The listing builds one solid part. Answer for the finished solid, in the listing's coordinates (mm). A direction names the side the tool comes from. Coordinates: 2 decimals unless noted, no trailing zeros. Loops run counter-clockwise (first coordinate to the right, second up) from the corner with the lowest first, then second, coordinate; pieces in that order, holes last. Notation, with made-up numbers: (58, 58) - (70, 58) arc R15 cw to (70, 73) - close; hole circle Ø9 at (-29, 86). An arc over 180 degrees is marked (long way). Return JSON: item names as keys, results as strings. Group by question number.
1. Each of these flat-tipped pins is pushed along its axis until it touches: P1, Ø3, axis at x = -6, y = 64, coming from the +Z side; P2, Ø1.5, axis at y = 56.5, z = -9, coming from the +X side; P3, Ø10.5, axis at x = -42, z = -24, coming from the +Y side; P4, Ø6, axis at x = 42, z = -6, coming from the +Y side. Where does it stop, or does it pass through?
2. Section D-D (x = -30) is taken. Write down the section's boundary in (y, z), and give its area (3 significant figures).
3. The mould has two halves that part along Y. Classify faces 4 (the face through (-38, 10, -15)), 5 (the face through (25, 51, -15)), 6 (the face through (-0.465, 27.507, -7.395)): pulls with the +Y half, pulls with the -Y half, needs draft (parallel to the pull), parting line crosses it, or undercut.
4. Section C-C (y = 42.5) is taken. Write down the section's boundary in (x, z).
5. Which of the six approach directions +Z, -Z, +X, -X, +Y, -Y give full straight-line access (tool end or side, diameter ignored) to faces 1 (the face through (-23.938, 25.702, -14.79)), 2 (the face through (23.938, 25.702, -14.79)), 3 (the face through (-39.381, 4.585, -21.992))?
6. Section A-A (z = -24) is taken. Write down the section's boundary in (x, y), and give its area (3 significant figures).
7. Section B-B (x = 42) is taken. Write down the section's boundary in (y, z), and give its area (3 significant figures).
8. Find the intervals of material crossed by line 1 along X through (y, z) = (6, -24); line 2 along Z through (x, y) = (42, 4.75); line 3 along Y through (x, z) = (0, -25.75), in increasing order.
```python
from build123d import *

# Parameters (mm, degrees)
EXTRUDE_1_DEPTH             = 30
SKETCH_2_R                  = 20
CUT_EXTRUDE_1_DEPTH         = 15
SKETCH_3_R                  = 5
CUT_EXTRUDE_2_DEPTH         = 109.397550478
FILLET_5_R                  = 6
SKETCH_4_R                  = 15
CUT_EXTRUDE_3_DEPTH         = 15
FILLET_6_R                  = 2
HOLE_WIZARD_M62_D           = 6.6
HOLE_WIZARD_M62_CSINK_D     = 8
HOLE_WIZARD_M62_CSINK_ANGLE = 90
PATTERN_LINEAR_1_COUNT      = 2
PATTERN_LINEAR_1_PITCH      = 18
PATTERN_LINEAR_1_COUNT_DIR2 = 2
PATTERN_LINEAR_1_PITCH_DIR2 = 84
FILLET_7_R                  = 3


with BuildPart() as part:
    # Эскиз1 → Бобышка-Вытянуть1 (new body)
    with BuildSketch(Plane.XY):
        with BuildLine():
            Line((0, 10), (0, 0))
            Line((0, 0), (50, 0))
            Line((50, 0), (50, 10))
            Line((50, 10), (10, 10))
            ThreePointArc((10, 10), (20.916500663, 19.219814537), (25, 32.912878475))
            Line((25, 32.912878475), (25, 70.000152367))
            ThreePointArc((25, 70.000152367), (17.67766953, 87.677821896), (0, 95.000152367))
            Line((0, 95.000152367), (0, 32.912878475))
            Line((0, 32.912878475), (0, 10))
        make_face()
    extrude_1 = extrude(amount=-EXTRUDE_1_DEPTH)

    # Зеркальное отражение1: Бобышка-Вытянуть1 across plane
    add(extrude_1.mirror(Plane(origin=(0, 95.000152367, -30), x_dir=(0, 0, 1), z_dir=(-1, 0, 0))))

    # Эскиз2 → Вырез-Вытянуть1 (cut)
    with BuildSketch(Plane.XY):
        with Locations((0, 70.000152367)):
            Circle(SKETCH_2_R)
    extrude(amount=-CUT_EXTRUDE_1_DEPTH, mode=Mode.SUBTRACT)

    # Эскиз3 → Вырез-Вытянуть2 (cut, through all)
    with BuildSketch(Plane.XY.offset(-15)):
        with Locations((0, 70.000152367)):
            Circle(SKETCH_3_R)
    extrude(amount=-CUT_EXTRUDE_2_DEPTH, mode=Mode.SUBTRACT)

    # Скругление5
    fillet_5_edges = [part.edges().sort_by_distance(p)[0] for p in [
        (10, 10, -15),
        (-10, 10, -15),
    ]]
    fillet(fillet_5_edges, radius=FILLET_5_R)

    # Эскиз4 → Вырез-Вытянуть3 (cut)
    with BuildSketch(Plane.XY):
        with Locations((0, 42.5)):
            Circle(SKETCH_4_R)
    extrude(amount=-CUT_EXTRUDE_3_DEPTH, mode=Mode.SUBTRACT)

    # Скругление6
    fillet_6_edges = [part.edges().sort_by_distance(p)[0] for p in [
        (10.644789814, 53.068275631, -7.5),
        (-10.644789814, 53.068275631, -7.5),
    ]]
    fillet(fillet_6_edges, radius=FILLET_6_R)

    # Зенковка для винта с полупотайной головкой M62 (through all)
    with Locations(Plane(origin=(42, 10, -24), x_dir=(1, 0, 0), z_dir=(0, 1, 0))):
        with Locations((0, 0)):
            hole_wizard_m62 = CounterSinkHole(HOLE_WIZARD_M62_D / 2, HOLE_WIZARD_M62_CSINK_D / 2, counter_sink_angle=HOLE_WIZARD_M62_CSINK_ANGLE)

    # Линейный массив1: Hole Wizard M62 2 × 2
    with Locations(*[(-j * PATTERN_LINEAR_1_PITCH_DIR2, 0, i * PATTERN_LINEAR_1_PITCH) for i in range(PATTERN_LINEAR_1_COUNT) for j in range(PATTERN_LINEAR_1_COUNT_DIR2) if (i, j) != (0, 0)]):
        add(hole_wizard_m62, mode=Mode.SUBTRACT)

    # Скругление7
    fillet_7_edges = [part.edges().sort_by_distance(p)[0] for p in [
        (50, 5, 0),
        (50, 5, -30),
        (-50, 5, 0),
        (-50, 5, -30),
    ]]
    fillet(fillet_7_edges, radius=FILLET_7_R)


solid = part.part
```
The answers:
{
 "1": {"P1": "stops at z = -15", "P2": "stops at x = 25", "P3": "stops at y = 10", "P4": "passes through"},
 "2": {"outline": "(0, -30) - (10, -30) - (10, 0) - (0, 0) - close", "area": "300 mm2"},
 "3": {"face 4": "pulls with the +Y half", "face 5": "needs draft", "face 6": "undercut"},
 "4": {"outline": "(-25, -30) - (25, -30) - (25, 0) - (15, 0) - (15, -15) - (-15, -15) - (-15, 0) - (-25, 0) - close"},
 "5": {"face 1": "+Z, -Z, -X", "face 2": "+Z, -Z, +X", "face 3": "+Y, -Y"},
 "6": {"outline": "(-50, 0) - (-45.3, 0) - (-45.3, 9.3) - (-46, 10) - (-50, 10) - close; (-38.7, 0) - (38.7, 0) - (38.7, 9.3) - (38, 10) - (25.98, 10) arc R6 cw to (20.95, 19.27) arc R25 ccw to (25, 32.91) - (25, 70) arc R25 ccw to (-25, 70) - (-25, 32.91) arc R25 ccw to (-20.95, 19.27) arc R6 cw to (-25.98, 10) - (-38, 10) - (-38.7, 9.3) - close; (45.3, 0) - (50, 0) - (50, 10) - (46, 10) - (45.3, 9.3) - close; hole circle Ø10 at (0, 70)", "area": "4,660 mm2"},
 "7": {"outline": "(0, -30) - (10, -30) - (10, -28) - (9.3, -27.3) - (0, -27.3) - close; (0, -20.7) - (9.3, -20.7) - (10, -20) - (10, -10) - (9.3, -9.3) - (0, -9.3) - close; (0, -2.7) - (9.3, -2.7) - (10, -2) - (10, 0) - (0, 0) - close", "area": "167 mm2"},
 "8": {"line 1": "x = -50 to -45.3, -38.7 to 38.7, 45.3 to 50", "line 2": "z = -30 to -27.3, -20.7 to -9.3, -2.7 to 0", "line 3": "y = 0 to 65, 75 to 95"}
}
